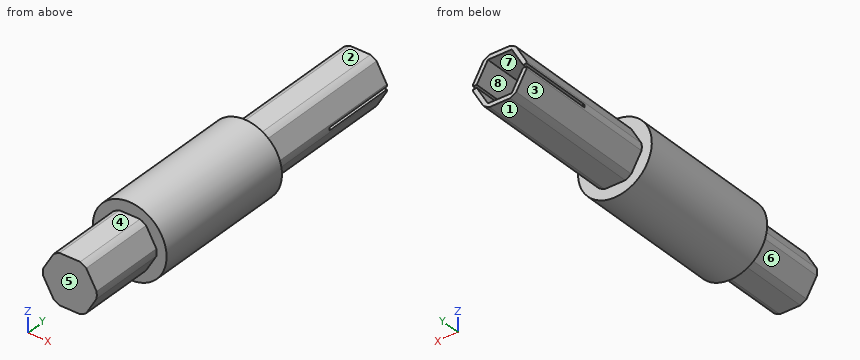
from build123d import *

# Parameters (mm, degrees)
BOSS_EXTRUDE1_DEPTH = 19.812
SKETCH2_R           = 9.5
BOSS_EXTRUDE2_DEPTH = 38.227
BOSS_EXTRUDE6_START = 76.327
BOSS_EXTRUDE6_DEPTH = 76.327
SKETCH6_W           = 13.85
SKETCH6_H           = 0.762
CUT_EXTRUDE1_DEPTH  = 19.05
CUT_EXTRUDE2_DEPTH  = 29.016999878


with BuildPart() as part:
    # Sketch1 → Boss-Extrude1 (new body)
    with BuildSketch(Plane(origin=(0, 0, 0), x_dir=(1, 0, 0), z_dir=(0, 1, 0))):
        with BuildLine():
            Line((6.86474929, 0.911505448), (4.221761519, 5.489294552))
            ThreePointArc((4.221761519, 5.489294552), (3.4625, 5.997225921), (2.642987771, 6.4008))
            Line((2.642987771, 6.4008), (-2.642987771, 6.4008))
            ThreePointArc((-2.642987771, 6.4008), (-3.4625, 5.997225921), (-4.221761519, 5.489294552))
            Line((-4.221761519, 5.489294552), (-6.86474929, 0.911505448))
            ThreePointArc((-6.86474929, 0.911505448), (-6.925, 0), (-6.86474929, -0.911505448))
            Line((-6.86474929, -0.911505448), (-4.221761519, -5.489294552))
            ThreePointArc((-4.221761519, -5.489294552), (-3.4625, -5.997225921), (-2.642987771, -6.4008))
            Line((-2.642987771, -6.4008), (2.642987771, -6.4008))
            ThreePointArc((2.642987771, -6.4008), (3.4625, -5.997225921), (4.221761519, -5.489294552))
            Line((4.221761519, -5.489294552), (6.86474929, -0.911505448))
            ThreePointArc((6.86474929, -0.911505448), (6.925, 0), (6.86474929, 0.911505448))
        make_face()
    extrude(amount=-BOSS_EXTRUDE1_DEPTH)

    # Sketch2 → Boss-Extrude2 (add)
    with BuildSketch(Plane(origin=(0, 0, 0), x_dir=(-1, 0, 0), z_dir=(0, -1, 0))):
        with Locations(Location((0, 0, 0), (0, 0, 90))):
            Circle(SKETCH2_R)
    extrude(amount=-BOSS_EXTRUDE2_DEPTH)

    # Sketch1_4 → Boss-Extrude6 (add)
    with BuildSketch(Plane(origin=(0, 0, 0), x_dir=(1, 0, 0), z_dir=(0, 1, 0)).offset(BOSS_EXTRUDE6_START)):
        with BuildLine():
            Line((6.86474929, 0.911505448), (4.221761519, 5.489294552))
            ThreePointArc((4.221761519, 5.489294552), (3.4625, 5.997225921), (2.642987771, 6.4008))
            Line((2.642987771, 6.4008), (-2.642987771, 6.4008))
            ThreePointArc((-2.642987771, 6.4008), (-3.4625, 5.997225921), (-4.221761519, 5.489294552))
            Line((-4.221761519, 5.489294552), (-6.86474929, 0.911505448))
            ThreePointArc((-6.86474929, 0.911505448), (-6.925, 0), (-6.86474929, -0.911505448))
            Line((-6.86474929, -0.911505448), (-4.221761519, -5.489294552))
            ThreePointArc((-4.221761519, -5.489294552), (-3.4625, -5.997225921), (-2.642987771, -6.4008))
            Line((-2.642987771, -6.4008), (2.642987771, -6.4008))
            ThreePointArc((2.642987771, -6.4008), (3.4625, -5.997225921), (4.221761519, -5.489294552))
            Line((4.221761519, -5.489294552), (6.86474929, -0.911505448))
            ThreePointArc((6.86474929, -0.911505448), (6.925, 0), (6.86474929, 0.911505448))
        make_face()
    extrude(amount=-BOSS_EXTRUDE6_DEPTH)

    # Sketch6 → Cut-Extrude1 (cut)
    with BuildSketch(Plane(origin=(0, 76.327, 0), x_dir=(1, 0, 0), z_dir=(0, 1, 0))):
        Rectangle(SKETCH6_W, SKETCH6_H)
    extrude(amount=-CUT_EXTRUDE1_DEPTH, mode=Mode.SUBTRACT)

    # Sketch7 → Cut-Extrude2 (cut)
    with BuildSketch(Plane(origin=(0, 76.327, 0), x_dir=(1, 0, 0), z_dir=(0, 1, 0))):
        Polygon((3.079586336, 5.334), (-3.079586336, 5.334), (-6.159172672, 0), (-3.079586336, -5.334), (3.079586336, -5.334), (6.159172672, 0), align=None)
    extrude(amount=-CUT_EXTRUDE2_DEPTH, mode=Mode.SUBTRACT)


solid = part.part
Part model, mm, in its own coordinate system. Face numbers are marked on the shaded views. A direction names the side the tool comes from. Round coordinates to 2 decimals unless told otherwise and drop trailing zeros. Order: outer loops, then holes, each group sorted by start corner. A loop starts at its lowest first (then second) coordinate and runs counter-clockwise, first axis right, second up. Notation, with made-up numbers: (10, 25) -> (17, 25) arc R15 cw to (17, 37) -> close; hole circle Ø10 at (-24.5, 34.5). An arc over 180 degrees is marked (long way). Put each result on its own line as item: value.
Q1. Band-saw the part on B-B (x = 0). Give the cut face in (y, z), and give its area (3 significant figures).
From the geometry:
outline: (-19.81, -6.4) -> (0, -6.4) -> (0, -9.5) -> (38.23, -9.5) -> (38.23, -6.4) -> (76.33, -6.4) -> (76.33, -5.33) -> (47.31, -5.33) -> (47.31, 5.33) -> (76.33, 5.33) -> (76.33, 6.4) -> (38.23, 6.4) -> (38.23, 9.5) -> (0, 9.5) -> (0, 6.4) -> (-19.81, 6.4) -> close
area: 1,160 mm2
Q2. Tool access for the marked faces 1, 2, 3 and 4: list every direction of +Z, -Z, +X, -X, +Y, -Y with a clear straight run to the whole face (end or side of a thin tool).
From the geometry:
face 1: -Z, +X, -X, +Y
face 2: +Z, +X, -X, +Y
face 3: -Z, -X, +Y
face 4: +Z, +X, -X, -Y
Q3. Pull direction Z, two halves, no side cores. Call the marked faces 5, 6, 7 and 8: pulls with the +Z half, pulls with the -Z half, needs draft (parallel to the pull), parting line crosses it, or undercut.
From the geometry:
face 5: needs draft
face 6: pulls with the -Z half
face 7: undercut
face 8: undercut
Q4. Pin check, flat tips, straight feed: pin 1 Ø1.6 at (x, y) = (-0.5, -11) entering from +Z; pin 2 Ø1.1 at (x, y) = (-6.5, 65.5) entering from -Z; pin 3 Ø1.8 at (x, y) = (0, 66.5) entering from -Z. Stop position of each tip, or through.
From the geometry:
pin 1: stops at z = 6.4
pin 2: stops at z = -2.5
pin 3: stops at z = -6.4
Q5. Wall check: line 1 (Z direction, x = 0, y = 66); line 2 (Y direction, x = -7, z = 2); line 3 (Z direction, x = -3.75, y = 63). Give the ranges that are in metal, low to high. Write a range as [from, to].
From the geometry:
line 1: z = [-6.4, -5.33], [5.33, 6.4]
line 2: y = [0, 38.23]
line 3: z = [-5.82, -4.17], [4.17, 5.82]
Q6. Band-saw the part on C-C (y = 16). Give the cut face in (x, z), and give its area (3 significant figures).
From the geometry:
outline: circle Ø19 at (0, 0)
area: 284 mm2
